Autodesk Inventor part; units mm, degrees
ref_plane "YZ Plane" through (0, 0, 0) normal (1, 0, 0) x (0, 1, 0)
ref_plane "XZ Plane" through (0, 0, 0) normal (0, 1, 0) x (-1, 0, 0)
ref_plane "XY Plane" through (0, 0, 0) normal (0, 0, 1) x (1, 0, 0)
sketch "Schizzo1" plane through (0, 0, 0) normal (0, 1, 0) x (-1, 0, 0)
  line L0 (0, 0) -> (130, 0)
  line L1 (130, 0) -> (130, -30)
  line L2 (130, -30) -> (0, -30)
  line L3 (0, -30) -> (0, 0)
  dimension "d0" = 30
  dimension "d1" = 130
extrude "Estrusione1" add sketch "Schizzo1" along normal blind 10
sketch "Schizzo2" plane through (0, 10, 0) normal (0, 1, 0) x (1, 0, 0)
  line L0 (-185.4023, 5) -> (-60, 5)
  line L1 (-60, 5) -> (-60, 25)
  line L2 (-60, 25) -> (-185.4023, 25)
  line L3 (-185.4023, 25) -> (-185.4023, 5)
  line L4 (-130, 0) -> (0, 0)
  line L5 (-130, 30) -> (-130, 0)
  point P0 (-130, 25)
  point P1 (-130, 5)
  dimension "d4" = 20
  dimension "d5" = 5
  dimension "d6" = 70
extrude "Estrusione2" cut sketch "Schizzo2" against normal blind 5 contours L5 L2 L1 L0
sketch "Schizzo3" plane through (0, 5, 0) normal (0, 1, 0) x (1, 0, 0)
  circle A0 centre (-127, 15) radius 1.65
  circle A1 centre (-117, 15) radius 1.3
  circle A2 centre (-97, 15) radius 1.3
  circle A3 centre (-77, 15) radius 1.3
  circle A4 centre (-67, 15) radius 1.65
  line L0 (-130, 0) -> (0, 0)
  line L1 (-130, 5) -> (-130, 25)
  line L2 (-145.516, 5) -> (-124, 5)
  line L3 (-124, 5) -> (-124, 25)
  line L4 (-124, 25) -> (-145.516, 25)
  line L5 (-145.516, 25) -> (-145.516, 5)
  line L6 (-60, 5) -> (-130, 5)
  line L7 (-70, 5) -> (-43.6658, 5)
  line L8 (-43.6658, 5) -> (-43.6658, 25)
  line L9 (-43.6658, 25) -> (-70, 25)
  line L10 (-70, 25) -> (-70, 5)
  dimension "d9" = 3.3
  dimension "d10" = 2.6
  dimension "d11" = 2.6
  dimension "d12" = 2.6
  dimension "d13" = 3.3
  dimension "d14" = 15
  dimension "d15" = 63
  dimension "d16" = 60
  dimension "d18" = 10
  dimension "d19" = 0
  dimension "d20" = 0
  dimension "d21" = 0
  dimension "d22" = 40
  dimension "d23" = 20
  dimension "d39" = 6
  dimension "d40" = 0
  dimension "d41" = 20
  dimension "d42" = 0
  dimension "d43" = 20
  dimension "d44" = 54
extrude "Estrusione3" cut sketch "Schizzo3" along normal through all both and the other way through all contours A0 | A1 | A2 | A3 | A4
sketch "Schizzo4" plane through (0, 10, 0) normal (0, 1, 0) x (1, 0, 0)
  circle A0 centre (-33.5752, 8) radius 1.25
  circle A1 centre (-19.5752, 8) radius 1.25
  circle A2 centre (-19.5752, 22) radius 1.25
  circle A3 centre (-33.5752, 22) radius 1.25
  line L0 (-130, 0) -> (0, 0)
  dimension "d26" = 14
  dimension "d27" = 14
  dimension "d28" = 14
  dimension "d29" = 14
  dimension "d30" = 0
  dimension "d31" = 0
  dimension "d32" = 8
  dimension "d33" = 2.5
  dimension "d34" = 2.5
  dimension "d35" = 2.5
  dimension "d36" = 2.5
extrude "Estrusione4" cut sketch "Schizzo4" against normal through all
sketch "Schizzo5" plane through (0, 5, 0) normal (0, 1, 0) x (1, 0, 0)
  line L0 (-60, 5) -> (-130, 5)
  line L1 (-130, 25) -> (-60, 25)
  line L2 (-60, 5) -> (-70.5, 5)
  line L3 (-70.5, 5) -> (-70.5, 25)
  line L4 (-70.5, 25) -> (-60, 25)
  line L5 (-60, 25) -> (-60, 5)
  line L6 (-130, 30) -> (-130, 0)
  line L7 (-130, 5) -> (-123.5, 5)
  line L8 (-123.5, 5) -> (-123.5, 25)
  line L9 (-123.5, 25) -> (-130, 25)
  line L10 (-130, 25) -> (-130, 5)
  point P0 (0, 0)
  point P1 (-123.5, 5)
  point P2 (-123.5, 25)
  dimension "d45" = 6.5
  dimension "d46" = 53
extrude "Estrusione5" add sketch "Schizzo5" along normal blind 5 contours L0 L3 L1 L5 | L0 L6 L1 L8
sketch "Schizzo6" plane through (0, 0, 0) normal (0, -1, 0) x (1, 0, 0)
  circle A0 centre (-127, -15) radius 1.65
  circle A1 centre (-127, -15) radius 1.65
  circle A2 centre (-67, -15) radius 1.65
  circle A3 centre (-67, -15) radius 1.65
  point P0 (0, 0)
  dimension "d49" = 3.3
  dimension "d50" = 3.3
extrude "Estrusione6" cut sketch "Schizzo6" against normal blind 50
properties part number "prortezione penna correnti parassite"
Read the model definition and answer for the solid it produces. Units are mm, in the model's axes. A direction names the side the tool comes from. Coordinates: 2 decimals unless noted, no trailing zeros. Loops run counter-clockwise (first coordinate to the right, second up) from the corner with the lowest first, then second, coordinate; pieces in that order, holes last. Notation, with made-up numbers: (24, 26) - (33, 26) arc R14 ccw to (33, 32) - close; hole circle Ø7 at (41.25, 31.5). An arc over 180 degrees is marked (long way). Answer in a Markdown table with one row per item.
1. Find section A-A, the plane z = -15. Write down the section's boundary in (x, y), then the cut area to 3 significant figures.
Conclusion:
| item | result |
|---|---|
| outline | (-130, 0) - (-128.65, 0) - (-128.65, 10) - (-130, 10) - close; (-125.35, 0) - (-118.3, 0) - (-118.3, 5) - (-123.5, 5) - (-123.5, 10) - (-125.35, 10) - close; (-115.7, 0) - (-98.3, 0) - (-98.3, 5) - (-115.7, 5) - close; (-95.7, 0) - (-78.3, 0) - (-78.3, 5) - (-95.7, 5) - close; (-75.7, 0) - (-68.65, 0) - (-68.65, 10) - (-70.5, 10) - (-70.5, 5) - (-75.7, 5) - close; (-65.35, 0) - (0, 0) - (0, 10) - (-65.35, 10) - close |
| area | 930 mm² |
2. Find section C-C, the plane y = 7.5. Write down the section's boundary in (x, z), then the cut area to 3 significant figures.
Conclusion:
| item | result |
|---|---|
| outline | (-130, -30) - (0, -30) - (0, 0) - (-130, 0) - close; hole circle Ø3.3 at (-127, -15); hole (-123.5, -25) - (-70.5, -25) - (-70.5, -5) - (-123.5, -5) - close; hole circle Ø3.3 at (-67, -15); hole circle Ø2.5 at (-33.58, -22); hole circle Ø2.5 at (-33.58, -8); hole circle Ø2.5 at (-19.58, -22); hole circle Ø2.5 at (-19.58, -8) |
| area | 2,800 mm² |
3. Find section B-B, the plane x = -127. Write down the section's boundary in (y, z).
Conclusion:
| item | result |
|---|---|
| outline | (0, -30) - (10, -30) - (10, -16.65) - (0, -16.65) - close; (0, -13.35) - (10, -13.35) - (10, 0) - (0, 0) - close |
4. Straight lines are drawn through the part: line 1 (X direction, y = 3.2, z = -15); line 2 (X direction, y = 9, z = -15); line 3 (Z direction, x = -77, y = 3.65). For each, find the intervals that lie inside material, in ascending order.
Conclusion:
| item | result |
|---|---|
| line 1 | x = -130 to -128.65, -125.35 to -118.3, -115.7 to -98.3, -95.7 to -78.3, -75.7 to -68.65, -65.35 to 0 |
| line 2 | x = -130 to -128.65, -125.35 to -123.5, -70.5 to -68.65, -65.35 to 0 |
| line 3 | z = -30 to -16.3, -13.7 to 0 |
5. Which of the six approach directions +Z, -Z, +X, -X, +Y, -Y give full straight-line access (tool end or side, diameter ignored) to faces 4 (the face through (-18.42, 5.07, -21.52)), 5 (the face through (-97, 5, -13))?
Conclusion:
| item | result |
|---|---|
| face 4 | +Y, -Y |
| face 5 | +Y |
6. Find section D-D, the plane z = -8. Write down the section's boundary in (x, y).
Conclusion:
| item | result |
|---|---|
| outline | (-130, 0) - (-34.83, 0) - (-34.83, 10) - (-70.5, 10) - (-70.5, 5) - (-123.5, 5) - (-123.5, 10) - (-130, 10) - close; (-32.33, 0) - (-20.83, 0) - (-20.83, 10) - (-32.33, 10) - close; (-18.33, 0) - (0, 0) - (0, 10) - (-18.33, 10) - close |
7. Determine the mould class of faces 1 (the face through (-115.8, 2.5, -14.5)), 2 (the face through (-64, 0, -15)), 3 (the face through (-64, 5, 0)) for opening direction Z: +Z half, -Z half, draft (parallel to the pull), parting line (faces both ways), or undercut.
Conclusion:
| item | result |
|---|---|
| face 1 | undercut |
| face 2 | draft |
| face 3 | +Z half |
8. Given pin 1 (5 mm diameter, centred on x = -41, z = -25, fed in from -Y); pin 2 (6 mm diameter, centred on x = -92, z = -17, fed in from +Y), each flat-ended and moving along its own axis, determine where each tip first touches the part or whether it passes through.
Conclusion:
| item | result |
|---|---|
| pin 1 | stops at y = 0 |
| pin 2 | stops at y = 5 |
